Source: CAD feature listing. Evaluate the final solid. Frame: model axes, mm. Give positions to 0.01 mm unless a question says otherwise; leave off trailing zeros. Order: outer loops, then holes, each group sorted by start corner. A loop starts at its lowest first (then second) coordinate and runs counter-clockwise, first axis right, second up. Notation, with made-up numbers: M 88.25,87.5 L 130.25,87.5 A12 cw 130.25,97.5 Z; hole C 62,89 d4. An arc over 180 degrees is marked long. Answer as a JSON object with one key per item and string values. Group by question number.
1. Section query A-A (z = 12). Output: boundary loops of the cut face in (x, y).
2. Pull-direction query (Y, two-part tool) for faces 1 (the cylindrical face through (-0.48, 22.56, 0.07)), 2 (the cylindrical face through (-48.933, -1.769, -7.465)), 3 (the flat face through (-14, -10, -5)); classes: +Y half, -Y half, draft (parallel to the pull), parting line (faces both ways), or undercut.
3. Section query D-D (y = 42.5). Output: boundary loops of the cut face in (x, z).
4. Pin query (flat end, axial travel): P1, Ø1, axis at x = 32.5, y = -17.5, coming from the -Z side; P2, Ø6, axis at y = -20, z = 6, coming from the -X side; P3, Ø1.5, axis at x = -57.5, y = 20.5, coming from the +Z side. Return the tip coordinate at first contact, or that it passes through.
5. Section query B-B (x = -80). Output: boundary loops of the cut face in (y, z), plus the area to 3 significant figures.
6. Material intervals for L1, parallel to Y at x = -79, z = 16; L2, parallel to X at y = 33, z = 2; L3, parallel to Y at x = -33.5, z = 3, sorted ascending. Write a range as [from, to].
7. Section query C-C (z = -7). Output: boundary loops of the cut face in (x, y), plus the area to 3 significant figures.
from build123d import *

# Parameters (mm, degrees)
SKETCH_R           = 15
SKETCH_R_2         = 8
SKETCH_R_3         = 13
PAD_DEPTH          = 5
SKETCH001_R        = 10.95
POCKET_DEPTH       = 413.746593
POCKET_DEPTH_BACK  = 413.746593
POLARPATTERN_COUNT = 8
SKETCH002_R        = 8
SKETCH002_R_2      = 13
PAD001_DEPTH       = 10
SKETCH003_R        = 13
SKETCH003_R_2      = 8
PAD002_DEPTH       = 20


with BuildPart() as part:
    # Sketch → Pad (new body, symmetric)
    with BuildSketch(Plane.XY):
        with BuildLine():
            ThreePointArc((5.273855, -51.932903), (52.142702, -2.445125), (10.110599, 51.211481))
            Line((10.110599, 51.211481), (-74.964069, 68.007634))
            ThreePointArc((-74.964069, 68.007634), (-100.516168, 58.471439), (-103.492932, 31.360784))
            ThreePointArc((-97.367005, -37.768495), (-94.240703, -2.65539), (-103.492932, 31.360784))
            ThreePointArc((-97.367005, -37.768495), (-93.732228, -54.137264), (-78.181429, -60.407898))
            Line((-78.181429, -60.407898), (5.273855, -51.932903))
        make_face()
        Circle(SKETCH_R, mode=Mode.SUBTRACT)
        with Locations((-80, -42.5)):
            Circle(SKETCH_R_2, mode=Mode.SUBTRACT)
        with Locations((-80, 42.5)):
            Circle(SKETCH_R_3, mode=Mode.SUBTRACT)
    extrude(amount=PAD_DEPTH, both=True)

    # Sketch001 → Pocket (cut, two sides)
    with BuildSketch(Plane.XY) as pocket_sk:
        with Locations((33.5, 0)):
            Circle(SKETCH001_R)
    pocket = extrude(amount=-POCKET_DEPTH, mode=Mode.SUBTRACT) + extrude(pocket_sk.sketch, amount=POCKET_DEPTH_BACK, mode=Mode.SUBTRACT)

    # PolarPattern: Pocket ×8 about axis
    polarpattern_axis = Axis((0, 0, 0), (0, 0, 1))
    for i in range(1, POLARPATTERN_COUNT):
        add(pocket.rotate(polarpattern_axis, i * 360 / POLARPATTERN_COUNT), mode=Mode.SUBTRACT)

    # Sketch002 → Pad001 (join, symmetric)
    with BuildSketch(Plane.XY):
        with BuildLine():
            ThreePointArc((-74.964069, 68.007634), (-100.516168, 58.471439), (-103.492932, 31.360784))
            ThreePointArc((-97.367005, -37.768495), (-94.240703, -2.65539), (-103.492932, 31.360784))
            ThreePointArc((-97.367005, -37.768495), (-93.732228, -54.137264), (-78.181429, -60.407898))
            ThreePointArc((-78.181429, -60.407898), (-70.117222, -57.544291), (-64.286757, -51.280319))
            ThreePointArc((-64.286757, -51.280319), (-48.867416, -1.030474), (-55.469, 51.115686))
            ThreePointArc((-55.469, 51.115686), (-62.973981, 62.149801), (-74.964069, 68.007634))
        make_face()
        with Locations((-80, -42.5)):
            Circle(SKETCH002_R, mode=Mode.SUBTRACT)
        with Locations((-80, 42.5)):
            Circle(SKETCH002_R_2, mode=Mode.SUBTRACT)
    extrude(amount=PAD001_DEPTH, both=True)

    # Sketch003 → Pad002 (join, symmetric)
    with BuildSketch(Plane.XY):
        with BuildLine():
            ThreePointArc((-74.964069, 68.007634), (-100.516168, 58.471439), (-103.492932, 31.360784))
            ThreePointArc((-103.492932, 31.360784), (-59.483832, 26.528561), (-74.964069, 68.007634))
        make_face()
        with Locations((-80, 42.5)):
            Circle(SKETCH003_R, mode=Mode.SUBTRACT)
        with BuildLine():
            ThreePointArc((-97.367005, -37.768495), (-93.732228, -54.137264), (-78.181429, -60.407898))
            ThreePointArc((-78.181429, -60.407898), (-66.267772, -30.862736), (-97.367005, -37.768495))
        make_face()
        with Locations((-80, -42.5)):
            Circle(SKETCH003_R_2, mode=Mode.SUBTRACT)
    extrude(amount=PAD002_DEPTH, both=True)


solid = part.part
Answer sheet:
{
 "1": {"outline": "C -80,42.5 d52; C -80,-42.5 d36; hole C -80,42.5 d26; hole C -80,-42.5 d16"},
 "2": {"face 1": "undercut", "face 2": "parting line", "face 3": "draft"},
 "3": {"outline": "M -106,-20 L -93,-20 L -93,20 L -106,20 Z; M -67,-20 L -54,-20 L -54,-10 L -52.79,-10 L -52.79,-5 L -6.24,-5 L -6.24,5 L -52.79,5 L -52.79,10 L -54,10 L -54,20 L -67,20 Z; M 6.24,-5 L 30.31,-5 L 30.31,5 L 6.24,5 Z"},
 "4": {"P1": "z = -5", "P2": "x = -94.52", "P3": "z = 10"},
 "5": {"outline": "M -60.5,-20 L -50.5,-20 L -50.5,20 L -60.5,20 Z; M -34.5,-20 L -24.5,-20 L -24.5,-10 L 16.5,-10 L 16.5,-20 L 29.5,-20 L 29.5,20 L 16.5,20 L 16.5,10 L -24.5,10 L -24.5,20 L -34.5,20 Z; M 55.5,-20 L 68.5,-20 L 68.5,20 L 55.5,20 Z", "area": "2,660 mm^2"},
 "6": {"L1": "[-60.47, -50.44], [-34.56, -24.53], [16.52, 29.54], [55.46, 68.48]", "L2": "[-104.2, -88.87], [-71.13, -29.45], [-17.93, -10.94], [10.94, 17.93], [29.45, 40.45]", "L3": "[-55.87, -28.55], [-18.83, -10.95], [10.95, 18.83], [28.55, 59.82]"},
 "7": {"outline": "M -103.49,31.36 A100 cw -97.37,-37.77 A18 ccw -64.29,-51.28 A125 ccw -55.47,51.12 A26 ccw -74.96,68.01 A26 ccw Z; hole C -80,42.5 d26; hole C -80,-42.5 d16", "area": "4,780 mm^2"}
}
